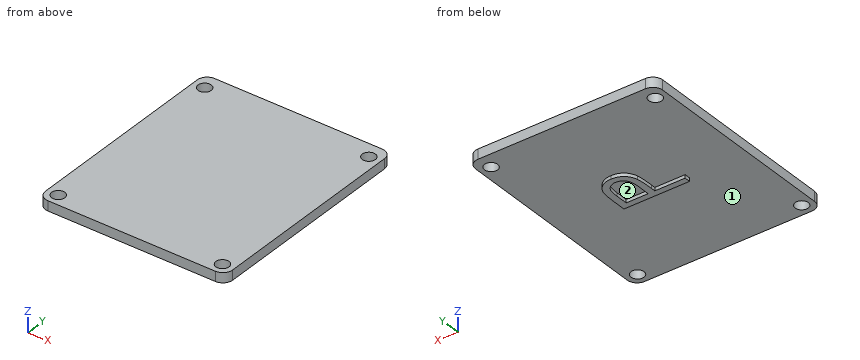
```python
from build123d import *

# Parameters (mm, degrees)
SKICA1_W                = 57
SKICA1_H                = 67
SKICA1_R                = 2
P_IDAT_VYSUNUT_M1_DEPTH = 3
P_IDAT_VYSUNUT_M2_DEPTH = 1
ZAOBLIT1_R              = 3


with BuildPart() as part:
    # Skica1 → Přidat vysunutím1 (new body)
    with BuildSketch(Plane.XY):
        with Locations((28.5, 33.5)):
            Rectangle(SKICA1_W, SKICA1_H)
        with Locations((3.5, 62.35016579)):
            Circle(SKICA1_R, mode=Mode.SUBTRACT)
        with Locations((53.5, 62.35016579)):
            Circle(SKICA1_R, mode=Mode.SUBTRACT)
        with Locations((53.5, 3.5)):
            Circle(SKICA1_R, mode=Mode.SUBTRACT)
        with Locations((3.5, 3.5)):
            Circle(SKICA1_R, mode=Mode.SUBTRACT)
    extrude(amount=P_IDAT_VYSUNUT_M1_DEPTH)

    # Skica2 → Přidat vysunutím2 (add)
    with BuildSketch(Plane(origin=(0, 0, 0), x_dir=(-1, 0, 0), z_dir=(0, 0, -1))):
        with BuildLine():
            Line((-37.970657991, 29.469714485), (-37.970657991, 33.391990126))
            add(Edge.make_bspline(
                [(-37.970657991, 33.391990126), (-37.970361441, 33.661766733), (-37.969793238, 34.178670691), (-37.952566119, 34.919899581), (-37.92955645, 35.593098048), (-37.897659918, 36.19681451), (-37.859965116, 36.732906499), (-37.80709632, 37.198948211), (-37.751894631, 37.598602818), (-37.695772308, 37.838068244), (-37.670177222, 37.947278587)],
                knots=[0, 0, 0, 0, 1.415646017, 2.712440637, 3.8905458, 4.950247383, 5.884950622, 6.709939814, 7.411656543, 8, 8, 8, 8], degree=3))
            add(Edge.make_bspline(
                [(-37.670177222, 37.947278587), (-37.632336028, 38.085526146), (-37.557545321, 38.358763633), (-37.407774038, 38.752501326), (-37.230082137, 39.12702996), (-37.027953627, 39.484021162), (-36.791438809, 39.8169729), (-36.53627201, 40.136984307), (-36.245963268, 40.432759), (-35.929669008, 40.708303209), (-35.591400822, 40.962981078), (-35.22501281, 41.176956538), (-34.841443644, 41.364050016), (-34.435480303, 41.51723294), (-34.006728651, 41.631146127), (-33.558235665, 41.715715192), (-33.089497036, 41.76963955), (-32.769150626, 41.774786619), (-32.606074658, 41.777406793)],
                knots=[0, 0, 0, 0, 0.999549623, 1.97554611, 2.93413192, 3.889860808, 4.833293765, 5.780583482, 6.742559327, 7.719844669, 8.705620613, 9.691528643, 10.674968152, 11.680406189, 12.713313868, 13.765869198, 14.862690416, 16, 16, 16, 16], degree=3))
            add(Edge.make_bspline(
                [(-32.606074658, 41.777406793), (-32.441630219, 41.774998651), (-32.119883568, 41.77028696), (-31.649181921, 41.713736758), (-31.199362549, 41.637564235), (-30.771422832, 41.520438221), (-30.367904143, 41.367034375), (-29.982639961, 41.187079788), (-29.622184693, 40.970031043), (-29.285229735, 40.720632016), (-28.971458808, 40.443194333), (-28.683145696, 40.13889183), (-28.421978048, 39.808953015), (-28.18737037, 39.454426455), (-27.984763059, 39.07185589), (-27.803292745, 38.667043584), (-27.650886684, 38.236470919), (-27.570714904, 37.938513696), (-27.529952863, 37.787022177)],
                knots=[0, 0, 0, 0, 1.121902311, 2.195077645, 3.232258892, 4.234102512, 5.217864754, 6.176164875, 7.132989551, 8.084763148, 9.034132444, 9.988522005, 10.94243251, 11.903244335, 12.886203696, 13.894208494, 14.929344452, 16, 16, 16, 16], degree=3))
            add(Edge.make_bspline(
                [(-27.529952863, 37.787022177), (-27.503327115, 37.661721699), (-27.44497524, 37.387118416), (-27.379389367, 36.934902646), (-27.325601784, 36.408121947), (-27.275406782, 35.808568661), (-27.248809706, 35.134844643), (-27.2175804, 34.388495093), (-27.202844998, 33.566994114), (-27.201913537, 32.994022793), (-27.201427222, 32.694874741)],
                knots=[0, 0, 0, 0, 0.601372724, 1.317943291, 2.144091499, 3.08771165, 4.142394186, 5.309582461, 6.595334295, 8, 8, 8, 8], degree=3))
            Line((-27.201427222, 32.694874741), (-27.201427222, 31.26458628))
            Line((-27.201427222, 31.26458628), (-17.970657991, 31.26458628))
            Line((-17.970657991, 31.26458628), (-17.970657991, 29.469714485))
            Line((-17.970657991, 29.469714485), (-37.970657991, 29.469714485))
        make_face()
        with BuildLine():
            Line((-35.91937594, 31.26458628), (-29.252709273, 31.26458628))
            Line((-29.252709273, 31.26458628), (-29.20863876, 34.766188844))
            add(Edge.make_bspline(
                [(-29.20863876, 34.766188844), (-29.208544615, 34.937161044), (-29.208362868, 35.267219352), (-29.231212915, 35.74398178), (-29.257239208, 36.186374829), (-29.296602466, 36.592734917), (-29.348201463, 36.964487883), (-29.412369977, 37.298422688), (-29.482131358, 37.599533869), (-29.59868532, 37.945903952), (-29.777898997, 38.335235337), (-30.038784485, 38.760550157), (-30.376749174, 39.118208289), (-30.755679044, 39.427140639), (-31.176087647, 39.677123759), (-31.628265809, 39.853476877), (-32.105514558, 39.962067848), (-32.431886932, 39.97562982), (-32.598061837, 39.982534998)],
                knots=[0, 0, 0, 0, 1.160746174, 2.240796558, 3.240300023, 4.169675897, 5.012224395, 5.787635701, 6.478238024, 7.109103438, 8.265591281, 9.382545711, 10.479929969, 11.588830844, 12.694575677, 13.785760505, 14.872603606, 16, 16, 16, 16], degree=3))
            add(Edge.make_bspline(
                [(-32.598061837, 39.982534998), (-32.758853186, 39.975319803), (-33.078486486, 39.96097689), (-33.546938864, 39.854373012), (-33.99399119, 39.675230054), (-34.411014182, 39.42692209), (-34.789110253, 39.125487049), (-35.118120247, 38.775412024), (-35.380842639, 38.375801415), (-35.556946227, 38.007170082), (-35.66004866, 37.677065259), (-35.734515791, 37.39175206), (-35.785866012, 37.067954947), (-35.835001767, 36.708750483), (-35.874664128, 36.314594731), (-35.902207185, 35.882982532), (-35.918157543, 35.415351195), (-35.918959975, 35.090720886), (-35.91937594, 34.922438844)],
                knots=[0, 0, 0, 0, 1.120540835, 2.227496496, 3.330685923, 4.466139262, 5.598993257, 6.692710361, 7.80064471, 8.921224235, 9.527843361, 10.209888745, 10.975318552, 11.811557897, 12.738105936, 13.73658638, 14.826690375, 16, 16, 16, 16], degree=3))
            Line((-35.91937594, 34.922438844), (-35.91937594, 31.26458628))
        make_face(mode=Mode.SUBTRACT)
    extrude(amount=P_IDAT_VYSUNUT_M2_DEPTH)

    # Zaoblit1
    zaoblit1_edges = [part.edges().sort_by_distance(p)[0] for p in [
        (0, 67, 1.5),
        (57, 67, 1.5),
        (57, 0, 1.5),
        (0, 0, 1.5),
    ]]
    fillet(zaoblit1_edges, radius=ZAOBLIT1_R)


solid = part.part
```
CAD build for the part. Positions are in the model's coordinates, mm. Face numbers are marked on the shaded views. Give positions to 0.01 mm unless a question says otherwise; leave off trailing zeros. Loops run counter-clockwise (first coordinate to the right, second up) from the corner with the lowest first, then second, coordinate; pieces in that order, holes last. Notation, with made-up numbers: (-31, 46) - (10, 46) arc R14 cw to (10, 56) - close; hole circle Ø6 at (1, -24). An arc over 180 degrees is marked (long way). Put each result on its own line as item: value.
Q1. Probe line 1 along Y through (x, z) = (3.5, 2.2); line 2 along Z through (x, y) = (44, 57); line 3 along Y through (x, z) = (21.5, -0.45). List the from-to ranges inside material, lowest first.
Filled in:
line 1: y = 0 to 1.5, 5.5 to 60.35, 64.35 to 67
line 2: z = 0 to 3
line 3: y = 29.47 to 31.26
Q2. Slice it at B-B (x = 41). Give the cut face in (y, z).
Filled in:
outline: (0, 0) - (67, 0) - (67, 3) - (0, 3) - close
Q3. Slice it at A-A (z = 1.6). Give the cut face in (x, y).
Filled in:
outline: (0, 3) arc R3 ccw to (3, 0) - (54, 0) arc R3 ccw to (57, 3) - (57, 64) arc R3 ccw to (54, 67) - (3, 67) arc R3 ccw to (0, 64) - close; hole circle Ø4 at (3.5, 3.5); hole circle Ø4 at (3.5, 62.35); hole circle Ø4 at (53.5, 3.5); hole circle Ø4 at (53.5, 62.35)
Q4. Slice it at C-C (y = 12.5). Give the cut face in (x, z), plus the area to 3 significant figures.
Filled in:
outline: (0, 0) - (57, 0) - (57, 3) - (0, 3) - close
area: 171 mm²
Q5. Mould opens along X. For the marked faces 1 and 2 say: pulls with the +X half, pulls with the -X half, needs draft (parallel to the pull), parting line crosses it, or undercut.
Filled in:
face 1: needs draft
face 2: undercut
Q6. Flat gauge pins, fed straight in: pin 1 (1.1 mm diameter, centred on y = 31.5, z = -0.5, fed in from +X); pin 2 (0.8 mm diameter, centred on y = 32, z = -0.5, fed in from -X); pin 3 (0.5 mm diameter, centred on x = 34, z = -0.5, fed in from +Y); pin 4 (0.5 mm diameter, centred on y = 30, z = -0.5, fed in from -X). Where does each tip first touch, or does it go through?
Filled in:
pin 1: stops at x = 57
pin 2: stops at x = 27.2
pin 3: stops at y = 41.68
pin 4: stops at x = 17.97
